Geometry: final body of the model. Coordinates: model frame, mm. Face numbers are marked on the shaded views. A direction names the side the tool comes from. Round coordinates to 2 decimals unless told otherwise and drop trailing zeros. Loops run counter-clockwise (first coordinate to the right, second up) from the corner with the lowest first, then second, coordinate; pieces in that order, holes last. Notation, with made-up numbers: (61.5, 6.25) - (70.5, 6.25) arc R30 cw to (70.5, 28.25) - close; hole circle Ø2 at (44, -2.5). An arc over 180 degrees is marked (long way). Answer as a JSON object with one key per item and string values. Group by question number.
Item 1: Draft query along X for the marked faces 4, 5 and 6. Return one class per face: released by +X, released by -X, zero draft, split by the parting line, or undercut.
Item 2: Reachability of the marked faces 1, 2 and 3 from +Z, -Z, +X, -X, +Y, -Y: full face, straight path, thin tool, end or side. Return the list, or none.
Item 3: Section A-A (x = -1). Return the cut outline in (y, z), plus the area to 3 significant figures.
Item 4: Line query: line 1 (Y direction, x = 19, z = 13.75); line 2 (X direction, y = 3, z = 14.5); line 3 (X direction, y = -4, z = 9). Output: solid intervals per line, ascending.
Item 5: First-contact query: pin 1 (0.6 mm diameter, centred on x = 41, y = -17.5, fed in from +Z); pin 2 (1.4 mm diameter, centred on x = -8.5, z = 19.5, fed in from +Y); pin 3 (3.5 mm diameter, centred on x = 46.5, z = 8, fed in from -Y); pin 4 (2 mm diameter, centred on x = 26.5, y = 0.5, fed in from -Z). Flat tips, straight axial feed; report the tip coordinate or a pass-through.
Item 6: Section B-B (y = -3). Return the cut outline in (x, z).
Item 7: Section C-C (z = 12.25). Return the cut outline in (x, y).
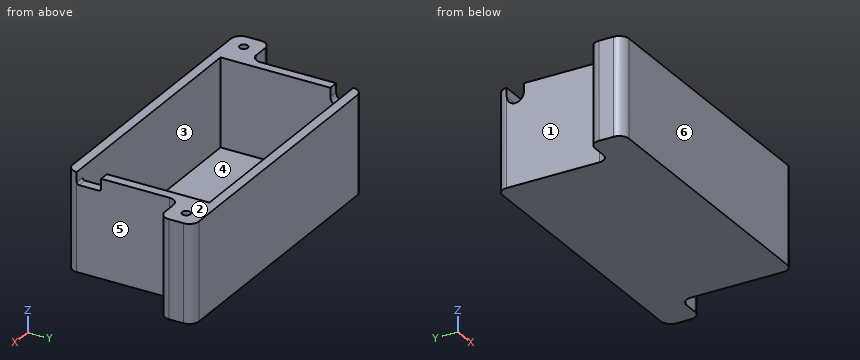
Autodesk Inventor part; units mm, degrees
ref_plane "YZ Plane" through (0, 0, 0) normal (1, 0, 0) x (0, 1, 0)
ref_plane "XZ Plane" through (0, 0, 0) normal (0, 1, 0) x (-1, 0, 0)
ref_plane "XY Plane" through (0, 0, 0) normal (0, 0, 1) x (1, 0, 0)
sketch "Эскиз1" plane through (0, 0, 0) normal (0, 0, 1) x (1, 0, 0)
  line L0 (-9.5803, -22.5479) -> (42.4197, -22.5479)
  line L1 (42.4197, -22.5479) -> (42.4197, 7.4521)
  line L2 (42.4197, 7.4521) -> (-9.5803, 7.4521)
  line L3 (-9.5803, 7.4521) -> (-9.5803, -22.5479)
extrude "Выдавливание1" add sketch "Эскиз1" along normal blind 2
sketch "Эскиз2" plane through (0, 0, 2) normal (0, 0, 1) x (1, 0, 0)
  line L0 (-9.5803, 7.4521) -> (-9.5803, -22.5479)
  line L1 (-9.5803, -22.5479) -> (42.4197, -22.5479)
  line L2 (-9.5803, 7.4521) -> (42.4197, 7.4521)
  line L3 (42.4197, 7.4521) -> (42.4197, -22.5479)
  line L4 (42.4197, -22.5479) -> (-9.5803, -22.5479)
  line L5 (-9.5803, -22.5479) -> (-9.5803, 7.4521)
  line L6 (42.4197, 7.4521) -> (-9.5803, 7.4521)
  line L7 (-9.5803, 7.4521) -> (-7.5803, 7.4521)
  line L8 (42.4197, -22.5479) -> (40.4197, -22.5479)
  line L9 (40.4197, -20.5479) -> (-7.5803, -20.5479)
  line L10 (-7.5803, -20.5479) -> (-7.5803, 5.4521)
  line L11 (-7.5803, 5.4521) -> (40.4197, 5.4521)
  line L12 (40.4197, 5.4521) -> (40.4197, -20.5479)
  point P0 (0, 0)
extrude "Выдавливание2" add sketch "Эскиз2" along normal blind 18
sketch "Эскиз6" plane through (0, 0, 0) normal (0, 0, -1) x (-1, 0, 0)
  line L0 (9.5803, -22.5479) -> (-42.4197, -22.5479)
  line L1 (9.5803, -22.5479) -> (16.5803, -22.5479)
  line L2 (16.5803, -22.5479) -> (16.5803, -15.5479)
  line L3 (16.5803, -15.5479) -> (9.5803, -15.5479)
  line L4 (9.5803, -15.5479) -> (9.5803, -22.5479)
  line L5 (-42.4197, 7.4521) -> (-49.4197, 7.4521)
  line L6 (-49.4197, 7.4521) -> (-49.4197, 0.4521)
  line L7 (-49.4197, 0.4521) -> (-42.4197, 0.4521)
  line L8 (-42.4197, 0.4521) -> (-42.4197, 7.4521)
  point P0 (0, 0)
  dimension "d22" = 7
  dimension "d23" = 7
  dimension "d24" = 7
  dimension "d25" = 7
extrude "Выдавливание5" add sketch "Эскиз6" against normal blind 20
sketch "Эскиз7" plane through (42.4197, -22.5479, 20) normal (1, 0, 0) x (0, 0, -1)
  line L0 (0, 2) -> (0, 28)
  line L1 (0, 2) -> (2.5, 2)
  line L2 (2.5, 2) -> (2.5, 7)
  line L3 (2.5, 7) -> (0, 7)
  line L4 (0, 7) -> (0, 2)
  point P0 (20, 22.5479)
  dimension "d28" = 2.5
  dimension "d29" = 5
extrude "Выдавливание6" cut sketch "Эскиз7" against normal blind 2
sketch "Эскиз8" plane through (-9.5803, 7.4521, 0) normal (-1, 0, 0) x (0, 0, 1)
  line L0 (2, -2) -> (20, -2)
  line L1 (20, -2) -> (18.25, -2)
  line L2 (16.5, -3.75) -> (16.5, -3.75)
  line L3 (18.25, -5.5) -> (20, -5.5)
  line L4 (20, -5.5) -> (20, -2)
  arc A0 (18.25, -2) -> (16.5, -3.75) centre (18.25, -3.75) ccw
  arc A1 (16.5, -3.75) -> (18.25, -5.5) centre (18.25, -3.75) ccw
  point P0 (0, -7.4521)
  point P1 (16.5, -5.5)
  point P2 (16.5, -2)
  dimension "d32" = 3.5
  dimension "d33" = 3.5
  dimension "d34" = 1.75
extrude "Выдавливание7" cut sketch "Эскиз8" against normal blind 2
fillet "Сопряжение1" radius 0.5 2 edges at (41.4197, -15.5479, 17.5) (41.4197, -20.5479, 17.5)
fillet "Сопряжение2" radius 2 8 edges at (42.4197, 0.4521, 10) (49.4197, 0.4521, 10) (49.4197, 7.4521, 10) (-9.5803, 7.4521, 10) (-16.5803, -22.5479, 10) (-16.5803, -15.5479, 10) (42.4197, -22.5479, 10) (-9.5803, -15.5479, 10)
sketch "Эскиз9" plane through (0, 0, 20) normal (0, 0, 1) x (1, 0, 0)
  circle A0 centre (-13.0803, -19.0479) radius 0.85
  point P0 (0, 0)
  point P1 (-16.5803, -17.5479)
  point P2 (-14.5803, -15.5479)
  dimension "d39" = 1.7
sketch "Эскиз10" plane through (0, 0, 20) normal (0, 0, 1) x (1, 0, 0)
  arc A0 (47.4197, 0.4521) -> (49.4197, 2.4521) centre (47.4197, 2.4521) ccw
  circle A1 centre (45.9197, 3.9521) radius 0.85
  point P0 (0, 0)
  dimension "d41" = 1.7
extrude "Выдавливание8" cut sketch "Эскиз9" against normal blind 15
extrude "Выдавливание9" cut sketch "Эскиз10" against normal blind 15
properties part number "Крышка Модуля БП"
Values:
{
 "1": {"face 4": "undercut", "face 5": "released by +X", "face 6": "zero draft"},
 "2": {"face 1": "+Z, -Z, -X, +Y", "face 2": "+Z, +X, -X, +Y, -Y", "face 3": "+Z"},
 "3": {"outline": "(-22.55, 0) - (7.45, 0) - (7.45, 20) - (5.45, 20) - (5.45, 2) - (-20.55, 2) - (-20.55, 20) - (-22.55, 20) - close", "area": "132 mm^2"},
 "4": {"line 1": "y = -22.55 to -20.55, 5.45 to 7.45", "line 2": "x = -9.58 to -7.58, 40.42 to 49.42", "line 3": "x = -9.58 to -7.58, 40.42 to 42.42"},
 "5": {"pin 1": "stops at z = 17.5", "pin 2": "stops at y = 7.44", "pin 3": "stops at y = 0.45", "pin 4": "stops at z = 0"},
 "6": {"outline": "(-9.58, 0) - (42.42, 0) - (42.42, 20) - (40.42, 20) - (40.42, 2) - (-7.58, 2) - (-7.58, 20) - (-9.58, 20) - close"},
 "7": {"outline": "(-16.58, -20.55) arc R2 ccw to (-14.58, -22.55) - (40.42, -22.55) arc R2 ccw to (42.42, -20.55) - (42.42, -1.55) arc R2 cw to (44.42, 0.45) - (47.42, 0.45) arc R2 ccw to (49.42, 2.45) - (49.42, 5.45) arc R2 ccw to (47.42, 7.45) - (-7.58, 7.45) arc R2 ccw to (-9.58, 5.45) - (-9.58, -13.55) arc R2 cw to (-11.58, -15.55) - (-14.58, -15.55) arc R2 ccw to (-16.58, -17.55) - close; hole circle Ø1.7 at (-13.08, -19.05); hole (-7.58, -20.55) - (40.42, -20.55) - (40.42, 5.45) - (-7.58, 5.45) - close; hole circle Ø1.7 at (45.92, 3.95)"}
}
